Can you work these out from the model? Positions are in its coordinate system, mm. Face numbers are marked on the shaded views. A direction names the side the tool comes from. Round coordinates to 2 decimals unless told otherwise and drop trailing zeros. Order: outer loops, then holes, each group sorted by start corner. A loop starts at its lowest first (then second) coordinate and runs counter-clockwise, first axis right, second up. Notation, with made-up numbers: (25, 18.5) - (38, 18.5) arc R14 cw to (38, 35.5) - close; hole circle Ø9 at (-11.75, 57). An arc over 180 degrees is marked (long way). Write item = value, one per line.
from build123d import *

# Parameters (mm, degrees)
SKETCH_1_R      = 3
SKETCH_1_R_2    = 1.75
EXTRUDE_1_DEPTH = 2
SKETCH_1_3_R    = 1.75
EXTRUDE_2_DEPTH = 30.6
FILLET_1_R      = 0.3


with BuildPart() as part:
    # Sketch 1 → Extrude 1 (new body)
    with BuildSketch(Plane.XY):
        Circle(SKETCH_1_R)
        Circle(SKETCH_1_R_2, mode=Mode.SUBTRACT)
        Circle(SKETCH_1_R_2)
    extrude(amount=EXTRUDE_1_DEPTH)

    # Sketch 1_3 → Extrude 2 (add)
    with BuildSketch(Plane.XY):
        Circle(SKETCH_1_3_R)
    extrude(amount=-EXTRUDE_2_DEPTH)

    # Fillet 1
    fillet_1_edges = [part.edges().sort_by_distance(p)[0] for p in [
        (-3, 0, 0),
        (-3, 0, 2),
        (-1.75, 0, -30.6),
        (-1.75, 0, 0),
    ]]
    fillet(fillet_1_edges, radius=FILLET_1_R)


solid = part.part
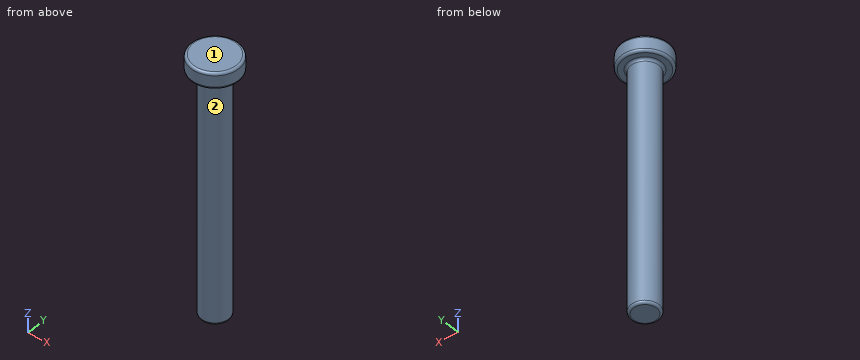
(1) If we section it at C-C (z = -19): Write out the boundary of the cut face in (x, y), plus the area to 3 significant figures.
Computed:
outline = circle Ø3.5 at (0, 0)
area = 9.62 mm^2
(2) If I drill on line 1 (Z direction, x = -2.5, y = -0.5); line 2 (Z direction, x = 1.5, y = 0); line 3 (X direction, y = 0.5, z = -23), over which ranges is the centre line in solid material (lowest first)? Write a range as from..to.
Computed:
line_1 = 0..2
line_2 = -30.6..2
line_3 = -1.68..1.68
(3) If we section it at A-A (y = 0): Write out the boundary of the cut face in (x, z).
Computed:
outline = (-3, 0.3) arc R0.3 ccw to (-2.7, 0) - (-2.05, 0) arc R0.3 cw to (-1.75, -0.3) - (-1.75, -30.3) arc R0.3 ccw to (-1.45, -30.6) - (1.45, -30.6) arc R0.3 ccw to (1.75, -30.3) - (1.75, -0.3) arc R0.3 cw to (2.05, 0) - (2.7, 0) arc R0.3 ccw to (3, 0.3) - (3, 1.7) arc R0.3 ccw to (2.7, 2) - (-2.7, 2) arc R0.3 ccw to (-3, 1.7) - close
(4) Will this pin go through, and if not, where does the flat tip stop? P1, Ø3, axis at x = 2, z = -16.5, coming from the -Y side.
Computed:
P1 = -1.68
(5) On a 3-axis mill with a long thin cutter (end or side, diameter ignored), from which of +Z, -Z, +X, -X, +Y, -Y can I reach the whole of each face in a straight line? I mean the marked faces 1 and 2. Say none if no direction works.
Computed:
face_1 = +Z, +X, -X, +Y, -Y
face_2 = -Z
